Autodesk Inventor part; units mm, degrees
ref_plane "YZ Plane" through (0, 0, 0) normal (1, 0, 0) x (0, 1, 0)
ref_plane "XZ Plane" through (0, 0, 0) normal (0, 1, 0) x (-1, 0, 0)
ref_plane "XY Plane" through (0, 0, 0) normal (0, 0, 1) x (1, 0, 0)
sketch "Sketch1" plane through (0, 0, 0) normal (0, 1, 0) x (-1, 0, 0)
  circle A0 centre (0, 0) radius 20
  dimension "d0" = 40
extrude "Extrusion1" add sketch "Sketch1" along normal blind 7
sketch "Sketch2" plane through (0, 7, 0) normal (0, 1, 0) x (1, 0, 0)
  circle A0 centre (0, 0) radius 40.2
  dimension "d3" = 80.4
extrude "Extrusion2" add sketch "Sketch2" along normal blind 4
sketch "Sketch3" plane through (0, 0, 0) normal (0, -1, 0) x (1, 0, 0)
  point P0 (0, 0)
  point P1 (0, 7)
  dimension "d6" = 7
hole "Hole1" at (0, 0, 7) direction (0, 1, 0) diameter 3.3 end through all
pattern_circular "Circular Pattern1" count 4 over 360 about axis through (0, -10, 0) along (0, 1, 0) of "Hole1"
sketch "Sketch4" plane through (0, 11, 0) normal (0, 1, 0) x (1, 0, 0)
  circle A0 centre (0, 0) radius 2.75
  dimension "d17" = 5.5
extrude "Extrusion3" cut sketch "Sketch4" against normal up to surface (11 mm away)
sketch "Sketch5" plane through (0, 0, 0) normal (0, -1, 0) x (1, 0, 0)
  circle A0 centre (0, 0) radius 4
  dimension "d20" = 8
extrude "Extrusion4" cut sketch "Sketch5" against normal blind 1
sketch "Sketch6" plane through (0, 11, 0) normal (0, 1, 0) x (1, 0, 0)
  circle A0 centre (0, 0) radius 2.75
  circle A1 centre (-7, 0) radius 1.65
  circle A2 centre (0, 7) radius 1.65
  circle A3 centre (7, 0) radius 1.65
  circle A4 centre (0, -7) radius 1.65
  circle A5 centre (0, 0) radius 40.2
  circle A6 centre (0, -7) radius 2.85
  dimension "d23" = 5.7
extrude "Extrusion5" cut sketch "Sketch6" against normal blind 4 contours A6
pattern_circular "Circular Pattern2" count 4 over 360 about axis through (0, 11, 0) along (0, -1, 0) of "Extrusion5"
sketch "Sketch8" plane through (0, 11, 0) normal (0, 1, 0) x (1, 0, 0)
  line L0 (-14, -9) -> (14, -9)
  line L1 (14, -9) -> (14, 8)
  line L2 (14, 8) -> (-14, 8)
  line L3 (-14, 8) -> (-14, -9)
  circle A0 centre (7, 0) radius 2.85
  circle A1 centre (0, 7) radius 2.85
  circle A2 centre (-7, 0) radius 2.85
  circle A3 centre (0, -7) radius 2.85
  circle A4 centre (0, 0) radius 2.75
  circle A5 centre (0, 0) radius 40.2
  dimension "d29" = 17
  dimension "d30" = 28
  dimension "d31" = 7
  dimension "d32" = 7
  dimension "d33" = 2
hole "Hole2" at (-14, 11, 9) at (14, 11, 9) at (14, 11, -8) at (-14, 11, -8) direction (0, -1, 0) diameter 2.459 end through all
equation "\"d31\" = d32"
properties part number "table_2"
Design review of the part built by this model. Coordinates are the model's own, in mm. A direction names the side the tool comes from. Coordinates: 2 decimals unless noted, no trailing zeros. Loops run counter-clockwise (first coordinate to the right, second up) from the corner with the lowest first, then second, coordinate; pieces in that order, holes last. Notation, with made-up numbers: (1, 24) - (42, 24) arc R28 ccw to (42, 57) - close; hole circle Ø6 at (34, 24). An arc over 180 degrees is marked (long way). Use CSV: the item, a comma, the result in double quotes. Start each with the question number.
1. Mouldability with a two-part tool opening along X and no side actions: class faces 1 (the cylindrical face through (4.336, 3.451, 19.524)), 2 (the cylindrical face through (12.963, 5.423, 9.661)), 3 (the flat face through (8.4, 7, -18.4)) as released by +X, released by -X, zero draft, split by the parting line, or undercut.
2. For faces 4 (the flat face through (3, 1, 1)), 5 (the cylindrical face through (-8.65, 3.55, -0.07)), 6 (the flat face through (0, 7, -9)), list the 3-axis set-ups (+Z, -Z, +X, -X, +Y, -Y) from which the entire face can be reached by the end or side of a thin tool; tool diameter is ignored.
3. Add section A-A on y = 5.75. Count the separate pieces of the cut face and the enclosed holes in it, plus the area to 3 significant figures.
4. Add section B-B on x = 14. Give the boundary of the cut face in (y, z).
5. Add section C-C on z = 28. Give the boundary of the cut face in (x, y).
6. Add section D-D on x = -22.5. Give the boundary of the cut face in (y, z), plus the area to 3 significant figures.
7. To check wall thickness, follow probe 1 along Z at (x, y) = (0, 4); probe 2 along Z at (x, y) = (0, 9.9); probe 3 along X at (y, z) = (2.5, 9). State the ranges of each line that lie inside material, in increasing order.
8. Clearance check with flat-ended pins moving along their axes: pin 1 (5 mm diameter, centred on x = 0, z = -7, fed in from +Y); pin 2 (1 mm diameter, centred on y = 9, z = -17, fed in from -X); pin 3 (6 mm diameter, centred on x = -7, z = 30, fed in from -Y). State where each tip first meets the part, or that it passes through.
Resolved:
1,face 1,"split by the parting line"
1,face 2,"undercut"
1,face 3,"zero draft"
2,face 4,"-Y"
2,face 5,"+Y, -Y"
2,face 6,"+Y"
3,separate pieces,"1"
3,enclosed holes,"9"
3,area,"1,180 mm2"
4,outline,"(0, -14.28) - (7, -14.28) - (7, -37.68) - (11, -37.68) - (11, -9.23) - (0, -9.23) - close; (0, -6.77) - (11, -6.77) - (11, 7.77) - (0, 7.77) - close; (0, 10.23) - (11, 10.23) - (11, 37.68) - (7, 37.68) - (7, 14.28) - (0, 14.28) - close"
5,outline,"(-28.85, 7) - (28.85, 7) - (28.85, 11) - (-28.85, 11) - close"
6,outline,"(7, -33.31) - (11, -33.31) - (11, 33.31) - (7, 33.31) - close"
6,area,"267 mm2"
7,probe 1,"-20 to -8.65, -5.35 to -2.75, 2.75 to 5.35, 8.65 to 20"
7,probe 2,"-40.2 to -9.85, -4.15 to -2.75, 2.75 to 4.15, 9.85 to 40.2"
7,probe 3,"-17.86 to -15.23, -12.77 to 12.77, 15.23 to 17.86"
8,pin 1,"y = 7"
8,pin 2,"x = -36.66"
8,pin 3,"y = 7"
